Answer from the drawing. Dimensions are ordinates in mm from the lowest x, y and z of the part. Round coordinates to 2 decimals unless told otherwise and drop trailing zeros. Write each loop counter-clockwise with the first axis right and the second up, starting at its lowest first coordinate (ties: lowest second). Pieces come first, ordered by that corner, then holes. Notation, with made-up numbers: M 26,58 L 48,58 A31 cw 48,88 Z; hole C 72.5,64 d1. An arc over 180 degrees is marked long. One line per item, written item: value. Start each with the question number.
(1) Section B-B (y = 53) is taken. Determine the outline of the cut face in (x, z).
(2) Section A-A (z = 11) is taken. Determine the outline of the cut face in (x, y) (1 decimal).
(3) Given P1, Ø6, axis at x = 55.5, z = 19, coming from the -Y side; P2, Ø6, axis at y = 64, z = 6.5, coming from the -X side; P3, Ø5, axis at x = 12.5, z = 3.5, coming from the -Y side, each flat-ended and moving along its own axis, determine where each tip first touches the part or whether it passes through.
(4) Consider probe 1 along Y at (x, z) = (59, 13.75) (1 decimal); probe 2 along X at (y, z) = (58.5, 3.75) (1 decimal); probe 3 along Y at (x, z) = (37, 7). Determine where each line is inside the solid, lowest interval first.
(5) Section C-C (x = 56) is taken. Determine the outline of the cut face in (y, z).
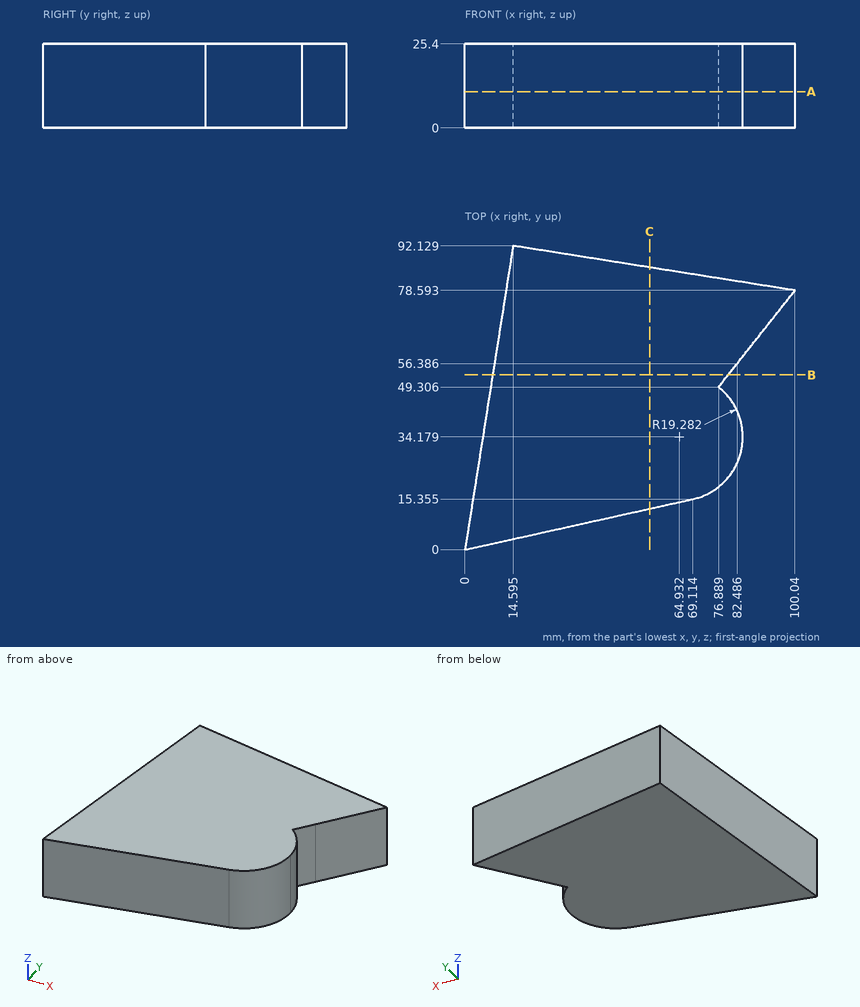
Recorded:
1. outline: M 8.4,0 L 79.81,0 L 79.81,25.4 L 8.4,25.4 Z
2. outline: M 0,0 L 69.1,15.4 A19.3 ccw 76.9,49.3 L 100,78.6 L 14.6,92.1 Z
3. P1: stops at y = 11.66
3. P2: stops at x = 9.66
3. P3: stops at y = 2.22
4. probe 1: y = 13.1 to 85.1
4. probe 2: x = 9.3 to 84.2
4. probe 3: y = 8.22 to 88.58
5. outline: M 12.44,0 L 85.57,0 L 85.57,25.4 L 12.44,25.4 Z
